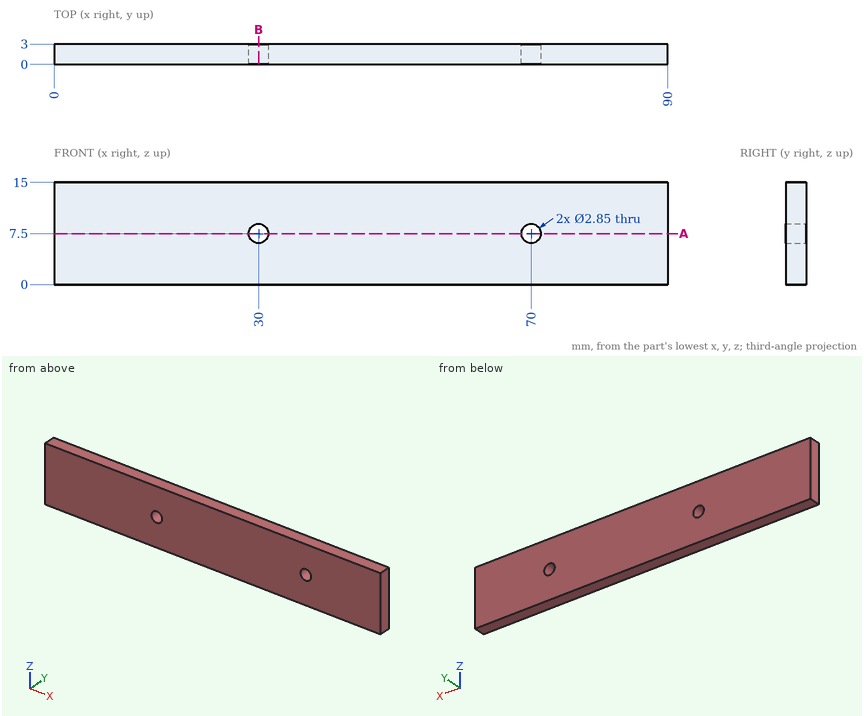
Design review of the part shown in the three views and the two pictorial views. Dimensions are in mm from the part's minimum x, y and z. Round coordinates to 2 decimals unless told otherwise and drop trailing zeros. Order: outer loops, then holes, each group sorted by start corner. A loop starts at its lowest first (then second) coordinate and runs counter-clockwise, first axis right, second up. Notation, with made-up numbers: (32.25, 41) - (61.25, 41) arc R14 cw to (61.25, 51) - close; hole circle Ø9 at (81, 45). An arc over 180 degrees is marked (long way). One line per question, with ' | ' between items.
Item 1: For P1, Ø2.5, axis at x = 70, z = 7.5, coming from the +Y side; P2, Ø5, axis at x = 43, z = 11.5, coming from the -Y side, all flat-tipped, find the tip position at first contact; note any pin that passes through.
Checks:
P1: through | P2: y = 0
Item 2: Take a section at A-A, the plane z = 7.5. Write out the cut boundary in (x, y) (3 decimals), then the cut area to 3 significant figures.
Checks:
outline: (0, 0) - (28.575, 0) - (28.575, 3) - (0, 3) - close; (31.425, 0) - (68.575, 0) - (68.575, 3) - (31.425, 3) - close; (71.425, 0) - (90, 0) - (90, 3) - (71.425, 3) - close | area: 253 mm²
Item 3: Take a section at B-B, the plane x = 30. Write out the cut boundary in (y, z) (3 decimals), then the cut area to 4 significant figures.
Checks:
outline: (0, 0) - (3, 0) - (3, 6.075) - (0, 6.075) - close; (0, 8.925) - (3, 8.925) - (3, 15) - (0, 15) - close | area: 36.45 mm²
Item 4: Wall thickness on line 1 (Z direction, x = 70, y = 1.85) (3 decimals); line 2 (Z direction, x = 31, y = 1.65); line 3 (X direction, y = 1.6, z = 6.75): over which ranges is each line inside the solid? List them lowest first. Write a range as [from, to].
Checks:
line 1: [0, 6.075], [8.925, 15] | line 2: [0, 6.48], [8.52, 15] | line 3: [0, 28.79], [31.21, 68.79], [71.21, 90]
